Can you work these out from the model? Positions are in its coordinate system, mm. A direction names the side the tool comes from. Round coordinates to 2 decimals unless told otherwise and drop trailing zeros. Order: outer loops, then holes, each group sorted by start corner. A loop starts at its lowest first (then second) coordinate and runs counter-clockwise, first axis right, second up. Notation, with made-up numbers: M 76,22 L 82,22 A30 ccw 82,58 Z; hole C 1.25,62 d5. An arc over 180 degrees is marked long. One line per question, with ' | ' between items.
```python
from build123d import *

# Parameters (mm, degrees)
BOSS_EXTRUDE1_DEPTH  = 3
M4_CLEARANCE_HOLE1_D = 4.5
SKETCH5_R            = 1.5875
CUT_EXTRUDE1_DEPTH   = 20
SKETCH7_R            = 1
CUT_EXTRUDE2_DEPTH   = 25.596747752


with BuildPart() as part:
    # Sketch2 → Boss-Extrude1 (new, symmetric)
    with BuildSketch(Plane.XY):
        with BuildLine():
            Line((13, 0), (13, -20))
            Line((13, -20), (7, -20))
            Line((7, -20), (7, -10.95445115))
            ThreePointArc((7, -10.95445115), (-11.401754251, 6.244997998), (13, 0))
        make_face()
    extrude(amount=BOSS_EXTRUDE1_DEPTH, both=True)

    # M4 Clearance Hole1 (through all)
    with Locations(Plane.XY.offset(3)):
        with Locations((0, 0)):
            Hole(M4_CLEARANCE_HOLE1_D / 2)

    # Sketch5 → Cut-Extrude1 (cut)
    with BuildSketch(Plane.XZ.offset(20)):
        with Locations(Location((10, 0, 0), (0, 0, 270))):
            Circle(SKETCH5_R)
    extrude(amount=-CUT_EXTRUDE1_DEPTH, mode=Mode.SUBTRACT)

    # Sketch7 → Cut-Extrude2 (cut, through all)
    with BuildSketch(Plane.XY.offset(3)):
        with Locations((-10, 0)):
            Circle(SKETCH7_R)
    extrude(amount=-CUT_EXTRUDE2_DEPTH, mode=Mode.SUBTRACT)


solid = part.part
```
(1) Please list where these lines run through material, in increasing order: probe 1 along Y at (x, z) = (0, -0.8); probe 2 along Y at (x, z) = (-1.5, 2.4); probe 3 along X at (y, z) = (-8, 0.7). Write a range as [from, to].
Final values:
probe 1: [-13, -2.25], [2.25, 13] | probe 2: [-12.91, -1.68], [1.68, 12.91] | probe 3: [-10.25, 8.58], [11.42, 13]
(2) If we section it at D-D on x = 10: Please give me the cut outline in (y, z).
Final values:
outline: M -20,-3 L 8.31,-3 L 8.31,3 L -20,3 L -20,1.59 L 0,1.59 L 0,-1.59 L -20,-1.59 Z
(3) If we section it at A-A on x = 0: Please give me the cut outline in (y, z).
Final values:
outline: M -13,-3 L -2.25,-3 L -2.25,3 L -13,3 Z; M 2.25,-3 L 13,-3 L 13,3 L 2.25,3 Z
(4) If we section it at C-C on y = -17.5: Please give me the cut outline in (x, z) (1 decimal).
Final values:
outline: M 7,-3 L 13,-3 L 13,3 L 7,3 Z; hole C 10,0 d3.2
(5) If we section it at B-B on z = 0: Please give me the cut outline in (x, y).
Final values:
outline: M 7,-20 L 8.41,-20 L 8.41,0 L 11.59,0 L 11.59,-20 L 13,-20 L 13,0 A13 ccw long 7,-10.95 Z; hole C -10,0 d2; hole C 0,0 d4.5
(6) Will these pins go through, and if not, where does the flat tip stop? pin 1 Ø1.6 at (x, z) = (10, 0.5) entering from -Y; pin 2 Ø1.5 at (x, y) = (2, -0.5) entering from +Z; pin 3 Ø2.5 at (x, y) = (0, 0) entering from +Z; pin 4 Ø1.5 at (x, z) = (-7, -2.5) entering from +Y.
Final values:
pin 1: y = 0 | pin 2: z = 3 | pin 3: through | pin 4: y = 11.4
(7) On a 3-axis mill with a long thin cutter (end or side, diameter ignored), from which of +Z, -Z, +X, -X, +Y, -Y can I reach the whole of each face in a straight line? I mean faces 4 (the flat face through (10, 0, 0)), 5 (the flat face through (8.7, -20, 1.4)). Say none if no direction works.
Final values:
face 4: -Y | face 5: +Z, -Z, +X, -X, -Y
(8) Thinking about a two-plate mould opening in Z: for faces 1 (the flat face through (7, -16, 0)), 2 (the cylindrical face through (8.59, -10.14, -0.73)), 3 (the flat face through (3, 0, 3)), which applies, released by +Z, released by -Z, zero draft, split by the parting line, or undercut?
Final values:
face 1: zero draft | face 2: undercut | face 3: released by +Z
